Build history of the part. All positions in model axes, mm. A direction names the side the tool comes from. Coordinates: 2 decimals unless noted, no trailing zeros. Loops run counter-clockwise (first coordinate to the right, second up) from the corner with the lowest first, then second, coordinate; pieces in that order, holes last.
(1) Slice it at C-C (z = 5). Give the cut face in (x, y), and give its area (3 significant figures).
(2) Wall check: L1, parallel to X at y = 135.75, z = 0; L2, parallel to Z at x = 0, y = 134.25; L3, parallel to X at y = 140, z = -1.75. Give the ranges that are in metal, low to high.
(3) Slice it at B-B (x = 0). Give the cut face in (y, z).
(4) Tool access for faces 1 (the face through (2.435, 139.878, -0.767)), 2 (the face through (-5.525, 75.133, -3.131)): list every direction of +Z, -Z, +X, -X, +Y, -Y with a clear straight run to the whole face (end or side of a thin tool).
(5) Slice it at A-A (y = 136.5). Give the cut face in (x, z).
(6) Flat gauge pin, fed straight in: P1, Ø1.5, axis at x = -1, z = -0.5, coming from the +Y side. Where does the tip first touch, or does it go through?
(7) Two-plate mould, pull along Z, no slides. Class faces 3 (the face through (5.474, 75.133, -3.219)), 4 (the face through (0, 127, 0)), 5 (the face through (0, 75, 6.35)): pulls with the +Z half, pulls with the -Z half, needs draft (parallel to the pull), parting line crosses it, or undercut.
(8) Slice it at D-D (z = -4). Give the cut face in (x, y), and give its area (3 significant figures).
Autodesk Inventor part; units mm, degrees
ref_plane "YZ Plane" through (0, 0, 0) normal (1, 0, 0) x (0, 1, 0)
ref_plane "XZ Plane" through (0, 0, 0) normal (0, 1, 0) x (-1, 0, 0)
ref_plane "XY Plane" through (0, 0, 0) normal (0, 0, 1) x (1, 0, 0)
sketch "Sketch1" plane through (0, 0, 0) normal (0, 1, 0) x (-1, 0, 0)
  line L0 (-7.3323, 0) -> (-3.6662, 6.35)
  line L1 (-3.6662, 6.35) -> (3.6662, 6.35)
  line L2 (3.6662, 6.35) -> (7.3323, 0)
  line L3 (7.3323, 0) -> (3.6662, -6.35)
  line L4 (3.6662, -6.35) -> (-3.6662, -6.35)
  line L5 (-3.6662, -6.35) -> (-7.3323, 0)
  point P0 (0, 0)
  point P1 (0, 0)
  point P2 (-5.4993, 3.175)
  dimension "d0" = 12.7
extrude "Extrusion1" add sketch "Sketch1" along normal blind 152.4
sketch "Sketch2" plane through (0, 152.4, 0) normal (0, 1, 0) x (1, 0, 0)
  circle A0 centre (0, 0) radius 2.5527
  dimension "d3" = 5.1054
extrude "Extrusion2" cut sketch "Sketch2" against normal blind 25.4
properties part number "INDEX_009_6inHex" material "Aluminum 6061"
Response values:
1. outline: (-4.45, 0) - (4.45, 0) - (4.45, 152.4) - (-4.45, 152.4) - close
1. area: 1,360 mm2
2. L1: x = -7.33 to -2.55, 2.55 to 7.33
2. L2: z = -6.35 to -2.55, 2.55 to 6.35
2. L3: x = -6.32 to -1.86, 1.86 to 6.32
3. outline: (0, -6.35) - (152.4, -6.35) - (152.4, -2.55) - (127, -2.55) - (127, 2.55) - (152.4, 2.55) - (152.4, 6.35) - (0, 6.35) - close
4. face 1: +Y
4. face 2: -Z, -X, +Y, -Y
5. outline: (-7.33, 0) - (-3.67, -6.35) - (3.67, -6.35) - (7.33, 0) - (3.67, 6.35) - (-3.67, 6.35) - close; hole circle Ø5.11 at (0, 0)
6. P1: stops at y = 127
7. face 3: pulls with the -Z half
7. face 4: undercut
7. face 5: pulls with the +Z half
8. outline: (-5.02, 0) - (5.02, 0) - (5.02, 152.4) - (-5.02, 152.4) - close
8. area: 1,530 mm2
